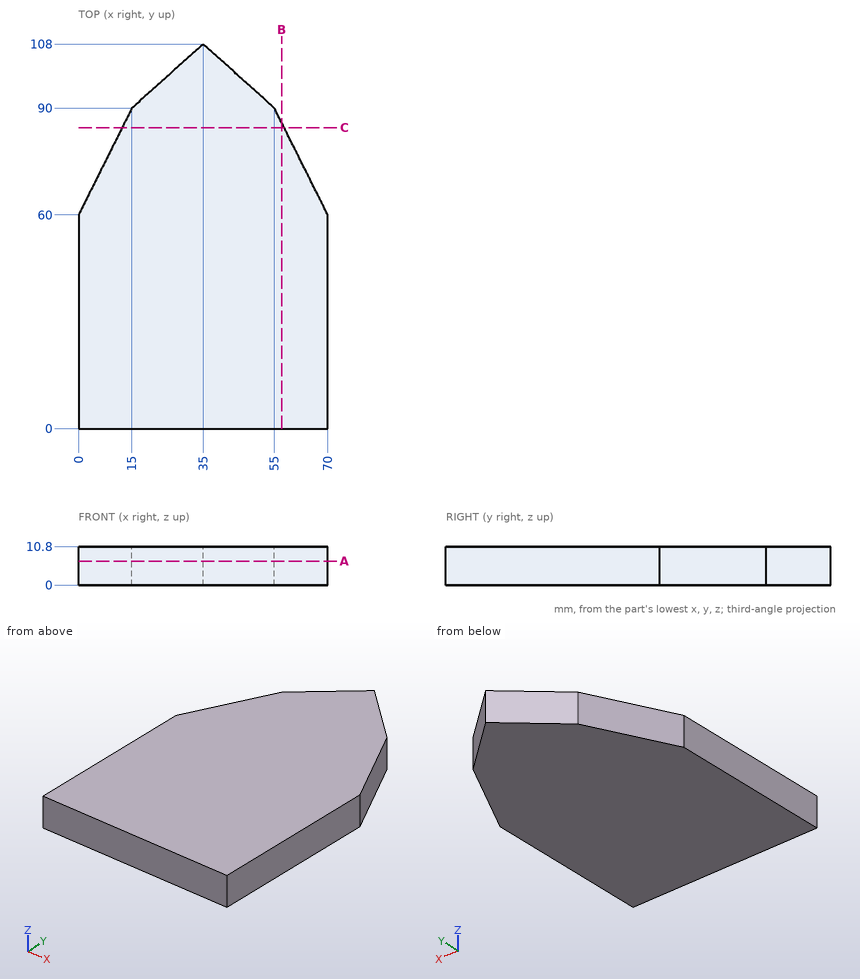
Geometry: see drawing. Coordinates: mm, zero at the bounding-box minimum. Coordinates: 2 decimals unless noted, no trailing zeros. Loops run counter-clockwise (first coordinate to the right, second up) from the corner with the lowest first, then second, coordinate; pieces in that order, holes last.
Q1. Cut plane A-A (z = 6.75). Output: boundary loops of the cut face in (x, y), then the cut area to 3 significant figures.
Q2. Material intervals for line 1 (X direction, y = 73, z = 6); line 2 (Y direction, x = 5, z = 2.5); line 3 (Y direction, x = 46, z = 7.75), sorted ascending.
Q3. Contact query for flat-ended pins moving along their axis: pin 1 (6 mm diameter, centred on y = 70, z = 5, fed in from -X); pin 2 (2 mm diameter, centred on x = 41.5, z = 6, fed in from +Y); pin 3 (5 mm diameter, centred on y = 87, z = 8, fed in from -X). Output: stop coordinate, or through.
Q4. Cut plane B-B (x = 57). Output: boundary loops of the cut face in (y, z).
Q5. Cut plane C-C (y = 84.5). Output: boundary loops of the cut face in (x, z).
Working result:
1. outline: (0, 0) - (70, 0) - (70, 60) - (55, 90) - (35, 108) - (15, 90) - (0, 60) - close
1. area: 6,210 mm2
2. line 1: x = 6.5 to 63.5
2. line 2: y = 0 to 70
2. line 3: y = 0 to 98.1
3. pin 1: stops at x = 3.5
3. pin 2: stops at y = 103.05
3. pin 3: stops at x = 12.25
4. outline: (0, 0) - (86, 0) - (86, 10.8) - (0, 10.8) - close
5. outline: (12.25, 0) - (57.75, 0) - (57.75, 10.8) - (12.25, 10.8) - close
